Check sheet for the drawn part. Datum: minimum x, y, z corner. Units: mm. Give positions to 0.01 mm unless a question says otherwise; leave off trailing zeros. Order: outer loops, then holes, each group sorted by start corner. A loop starts at its lowest first (then second) coordinate and runs counter-clockwise, first axis right, second up. Notation, with made-up numbers: (75, 29) -> (108, 29) arc R24 cw to (108, 63) -> close; hole circle Ø8 at (4.25, 23). An arc over 180 degrees is marked (long way). One line per question, with ' | ' between items. Start each with the question number.
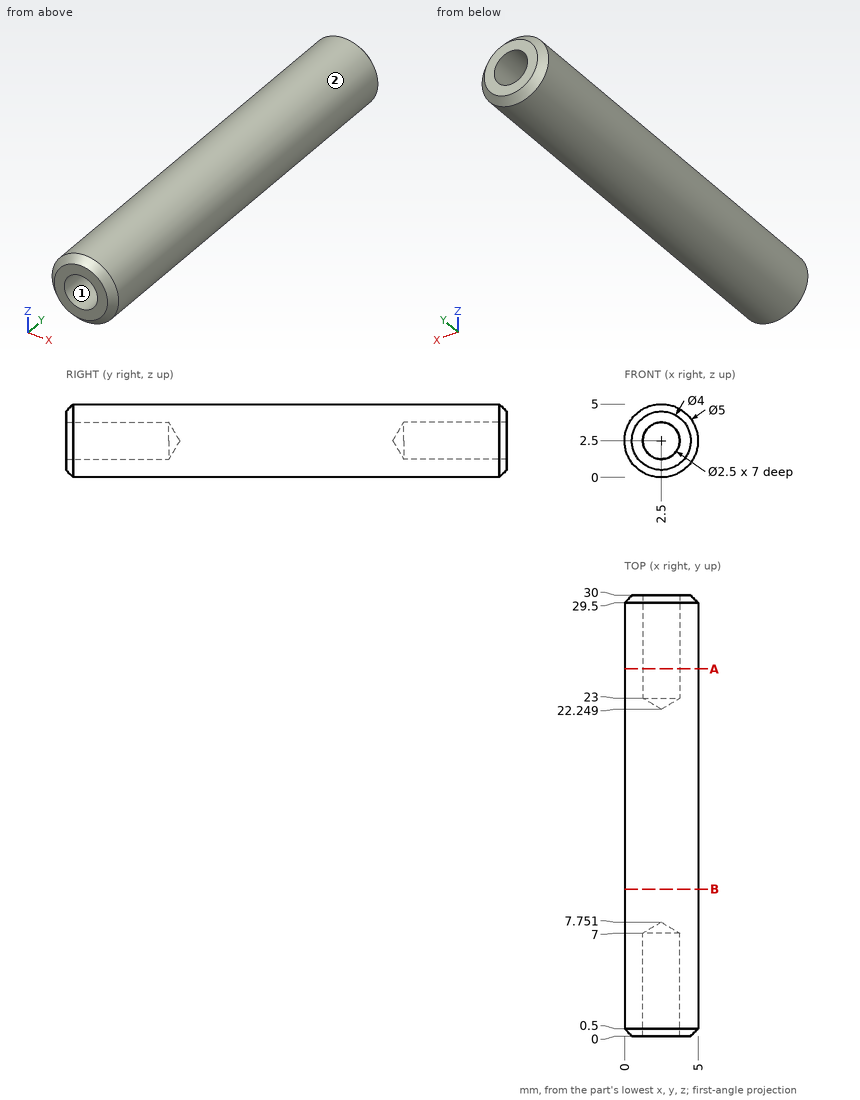
1. Cross-section at B-B on y = 10. Record the boundary of the cut face in (x, z), and give its area (3 significant figures).
2. Cross-section at A-A on y = 25. Record the boundary of the cut face in (x, z), and give its area (3 significant figures).
3. Go/stop test with a flat-tipped pin: pin 1 (1.5 mm diameter, centred on y = 25.5, z = 4.5, fed in from +X) (3 decimals). Record where the tip stops, or that it passes through.
4. Mould release check, pull along X, two halves, no side actions. Record for the marked faces 1 and 2: +X half, -X half, draft (parallel to the pull), parting line (faces both ways), or undercut.
5. Scan lines: probe 1 along X at (y, z) = (4.5, 2.55); probe 2 along Z at (x, y) = (1.7, 27); probe 3 along Z at (x, y) = (2.95, 23.25). Record each from-to range of solid material in increasing order.
Response values:
1) outline: circle Ø5 at (2.5, 2.5) | area: 19.6 mm²
2) outline: circle Ø5 at (2.5, 2.5); hole circle Ø2.5 at (2.5, 2.5) | area: 14.7 mm²
3) pin 1: stops at x = 4.665
4) face 1: undercut | face 2: parting line
5) probe 1: x = 0 to 1.25, 3.75 to 5 | probe 2: z = 0.13 to 1.54, 3.46 to 4.87 | probe 3: z = 0.04 to 1.33, 3.67 to 4.96
